from build123d import *

# Parameters (mm, degrees)
ESQUISSE1_R        = 1.5
ESQUISSE1_R_2      = 11
BOSS_EXTRU_1_DEPTH = 5


with BuildPart() as part:
    # Esquisse1 → Boss.-Extru.1 (new body)
    with BuildSketch(Plane(origin=(0, 0, 0), x_dir=(1, 0, 0), z_dir=(0, 1, 0))):
        with BuildLine():
            Line((-97.415, -97.415), (0, -97.415))
            Line((0, -97.415), (0, -37.415))
            ThreePointArc((0, -37.415), (-27.386127875, -26.569759474), (-39.921798557, 0.085))
            Line((-39.921798557, 0.085), (-147.415, 0.085))
            Line((-147.415, 0.085), (-147.415, -47.415))
            Line((-147.415, -47.415), (-97.415, -47.415))
            Line((-97.415, -47.415), (-97.415, -97.415))
        make_face()
        with Locations(Location((-72.415, -92.415, 0), (0, 0, 270))):
            Circle(ESQUISSE1_R, mode=Mode.SUBTRACT)
        with Locations(Location((-48.43544943, -69.915, 0), (0, 0, 270))):
            Circle(ESQUISSE1_R_2, mode=Mode.SUBTRACT)
        with Locations(Location((-142.415, -22.415, 0), (0, 0, 270))):
            Circle(ESQUISSE1_R, mode=Mode.SUBTRACT)
        with Locations(Location((-92.415, -42.415, 0), (0, 0, 270))):
            Circle(ESQUISSE1_R, mode=Mode.SUBTRACT)
        with Locations(Location((-31.819805153, -29.234805153, 0), (0, 0, 270))):
            Circle(ESQUISSE1_R, mode=Mode.SUBTRACT)
    extrude(amount=BOSS_EXTRU_1_DEPTH)


solid = part.part
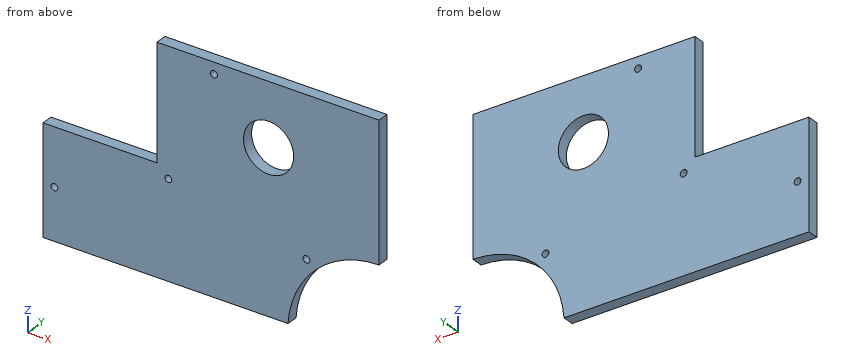
Here's how the part is built. I have some questions about the finished solid (model axes, mm). Round coordinates to 2 decimals unless told otherwise and drop trailing zeros. Loops run counter-clockwise (first coordinate to the right, second up) from the corner with the lowest first, then second, coordinate; pieces in that order, holes last. Notation, with made-up numbers: M 69.25,16 L 124.25,16 A23 ccw 124.25,54 Z; hole C 49,46.25 d9. An arc over 180 degrees is marked long. Write each question's results on one line, items separated by ' | '. Start each with the question number.
(1) I want a section at B-B (y = 1.15). Please give me the cut outline in (x, z) (3 decimals).
(2) I want a section at C-C (x = -54.5). Please give me the cut outline in (y, z) (3 decimals), then the cut area to 3 significant figures.
(3) If I drill on probe 1 along X at (y, z) = (1.95, 42.5) (3 decimals); probe 2 along X at (y, z) = (0.6, 82) (3 decimals); probe 3 along X at (y, z) = (1.7, 23.5) (3 decimals), over which ranges is the centre line in solid material (lowest first)? Write a range as from..to.
(4) Will these pins go through, and if not, where does the flat tip stop? P1, Ø1.5, axis at y = 3, z = 78, coming from the -X side (3 decimals); P2, Ø2.5, axis at x = -92.415, z = 42.415, coming from the +Y side.
(5) I want a section at D-D (x = -126.5). Please give me the cut outline in (y, z) (3 decimals).
(6) I want a section at A-A (z = 66.5). Please give me the cut outline in (x, y) (3 decimals).
Solved:
1) outline: M -147.415,-0.085 L -39.922,-0.085 A40 cw 0,37.415 L 0,97.415 L -97.415,97.415 L -97.415,47.415 L -147.415,47.415 Z; hole C -142.415,22.415 d3; hole C -92.415,42.415 d3; hole C -72.415,92.415 d3; hole C -48.435,69.915 d22; hole C -31.82,29.235 d3
2) outline: M 0,-0.085 L 5,-0.085 L 5,60.738 L 0,60.738 Z; M 0,79.092 L 5,79.092 L 5,97.415 L 0,97.415 Z | area: 396 mm²
3) probe 1: x = -147.415..-93.913, -90.917..0 | probe 2: x = -97.415..0 | probe 3: x = -147.415..-143.451, -141.379..-30.324
4) P1: stops at x = -97.415 | P2: passes through
5) outline: M 0,-0.085 L 5,-0.085 L 5,47.415 L 0,47.415 Z
6) outline: M -97.415,0 L -58.892,0 L -58.892,5 L -97.415,5 Z; M -37.979,0 L 0,0 L 0,5 L -37.979,5 Z
